```python
from build123d import *

# Parameters (mm, degrees)
F0_W     = 39.177138
F0_H     = 74.594855
F1_DEPTH = 33
F2_R     = 9.713505
F3_DEPTH = 92.75
F4_R     = 5


with BuildPart() as f1:
    # F0 (on Front) → F1 (new body)
    with BuildSketch(Plane.XZ):
        with Locations((19.588569, 37.297427)):
            Rectangle(F0_W, F0_H)
    extrude(amount=F1_DEPTH)

    # F2 (on face) → F3 (join)
    with BuildSketch(Plane.XZ.offset(33)):
        with Locations((20.775756, 39.572868)):
            Circle(F2_R)
    extrude(amount=F3_DEPTH)

    # F4
    f4_edges = [f1.edges().sort_by_distance(p)[0] for p in [
        (39.177138, 0, 37.297428),
        (19.588569, 0, 74.594855),
        (0, 0, 37.297428),
        (19.588569, 0, 0),
    ]]
    fillet(f4_edges, radius=F4_R)


solid = f1.part
```
Design review of the part built by this model. Coordinates are the model's own, in mm. A direction names the side the tool comes from. Give positions to 0.01 mm unless a question says otherwise; leave off trailing zeros. Order: outer loops, then holes, each group sorted by start corner. A loop starts at its lowest first (then second) coordinate and runs counter-clockwise, first axis right, second up. Notation, with made-up numbers: (73.5, 35.25) - (80.5, 35.25) arc R5 cw to (80.5, 44.25) - close; hole circle Ø8 at (67.5, 75.5). An arc over 180 degrees is marked (long way). Use a Markdown table: item, result. Add a question column.
(1) Wall thickness on probe 1 along Y at (x, z) = (18, 52.5); probe 2 along Y at (x, z) = (35.5, 59.5); probe 3 along X at (y, z) = (-48.5, 35): over which ranges is each line inside the solid? List them lowest first. Write a range as [from, to].
(2) Add section A-A on x = 32. Give the boundary of the cut face in (y, z), then the cut area to 3 significant figures.
(3) Add section B-B on z = 17.5. Give the boundary of the cut face in (x, y), then the cut area to 3 significant figures.
(4) Add section C-C on y = -95. Give the boundary of the cut face in (x, z), then the cut area to 3 significant figures.
(5) Machinability: for faces 1 (the face through (19, 0, 38)), 2 (the face through (19.511, -78.726, 49.204)), which of the approach directions +Z, -Z, +X, -X, +Y, -Y give a long, thin tool a straight path to every point of the face, cutting with its end or side? Answer none if there is none.
(6) Add section D-D on z = 47. Give the boundary of the cut face in (x, y), then the cut area to 3 significant figures.
(7) Clearance check with flat-ended pins moving along their axes: P1, Ø5, axis at x = 15.5, y = -73, coming from the -Z side; P2, Ø2, axis at y = -79.5, z = 44, coming from the -X side; P3, Ø5, axis at x = 27, z = 27, coming from the -Y side; P4, Ø12, axis at y = -42.5, z = 9, coming from the -X side. State where each tip first meets the part, or that it passes through.
Report:
| question | item | result |
|---|---|---|
| 1 | probe 1 | y = [-33, 0] |
| 1 | probe 2 | y = [-33, -0.18] |
| 1 | probe 3 | x = [12.21, 29.35] |
| 2 | outline | (-33, 0) - (-5, 0) arc R5 ccw to (0, 5) - (0, 69.59) arc R5 ccw to (-5, 74.59) - (-33, 74.59) - close |
| 2 | area | 2,450 mm² |
| 3 | outline | (0, -33) - (39.18, -33) - (39.18, -5) arc R5 ccw to (34.18, 0) - (5, 0) arc R5 ccw to (0, -5) - close |
| 3 | area | 1,280 mm² |
| 4 | outline | circle Ø19.43 at (20.78, 39.57) |
| 4 | area | 296 mm² |
| 5 | face 1 | +Z, -Z, +X, -X, +Y |
| 5 | face 2 | -Y |
| 6 | outline | (0, -33) - (14.52, -33) - (14.52, -125.75) - (27.04, -125.75) - (27.04, -33) - (39.18, -33) - (39.18, -5) arc R5 ccw to (34.18, 0) - (5, 0) arc R5 ccw to (0, -5) - close |
| 6 | area | 2,440 mm² |
| 7 | P1 | stops at z = 30.26 |
| 7 | P2 | stops at x = 11.69 |
| 7 | P3 | stops at y = -33 |
| 7 | P4 | passes through |
